```python
from build123d import *

# Parameters (mm, degrees)
SKETCH1_W           = 42
SKETCH1_H           = 42
BOSS_EXTRUDE1_DEPTH = 2
SKETCH2_R           = 2.225
SKETCH2_R_2         = 19
CUT_EXTRUDE1_DEPTH  = 2
FILLET1_R           = 5


with BuildPart() as part:
    # Sketch1 → Boss-Extrude1 (new body)
    with BuildSketch(Plane(origin=(0, 0, 0), x_dir=(1, 0, 0), z_dir=(0, 1, 0))):
        Rectangle(SKETCH1_W, SKETCH1_H)
    extrude(amount=BOSS_EXTRUDE1_DEPTH)

    # Sketch2 → Cut-Extrude1 (cut)
    with BuildSketch(Plane(origin=(0, 2, 0), x_dir=(1, 0, 0), z_dir=(0, 1, 0))):
        with Locations((-16, -16)):
            Circle(SKETCH2_R)
        with Locations((-16, 16)):
            Circle(SKETCH2_R)
        with Locations((16, 16)):
            Circle(SKETCH2_R)
        with Locations((16, -16)):
            Circle(SKETCH2_R)
        Circle(SKETCH2_R_2)
    extrude(amount=-CUT_EXTRUDE1_DEPTH, mode=Mode.SUBTRACT)

    # Fillet1
    fillet1_edges = [part.edges().sort_by_distance(p)[0] for p in [
        (-21, 1, 21),
        (-21, 1, -21),
        (21, 1, -21),
        (21, 1, 21),
    ]]
    fillet(fillet1_edges, radius=FILLET1_R)


solid = part.part
```
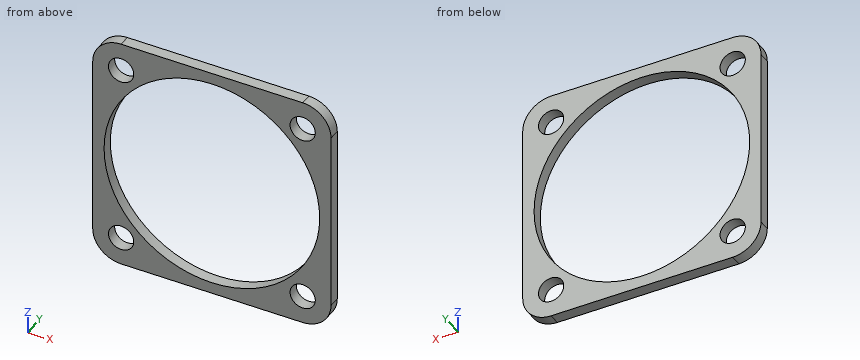
Geometry check sheet. Reference: the model listing, model coordinates, mm. Give positions to 0.01 mm unless a question says otherwise; leave off trailing zeros. Loops run counter-clockwise (first coordinate to the right, second up) from the corner with the lowest first, then second, coordinate; pieces in that order, holes last. Notation, with made-up numbers: M -37.75,85 L -11.75,85 A11 ccw -11.75,96 Z; hole C -12.75,16.25 d4. An arc over 180 degrees is marked long. Answer as CSV lines item,"result".
Item 1: Depth check by flat-ended pin: P1, Ø6, axis at x = 16, z = -16, coming from the +Y side; P2, Ø3.5, axis at x = 16, z = 16, coming from the -Y side. Enter the tip coordinate at first touch or a pass-through.
Values:
P1,"stops at y = 2"
P2,"passes through"
Item 2: Material ranges on line 1 (X direction, y = 1.3, z = 0); line 2 (X direction, y = 1.65, z = 16) (3 decimals), recorded low to high.
Values:
line 1,"x = -21 to -19, 19 to 21"
line 2,"x = -21 to -18.225, -13.775 to -10.247, 10.247 to 13.775, 18.225 to 21"
Item 3: Cross-section at B-B on x = 0. Record the cut outline in (y, z), and give its area (3 significant figures).
Values:
outline,"M 0,-21 L 2,-21 L 2,-19 L 0,-19 Z; M 0,19 L 2,19 L 2,21 L 0,21 Z"
area,"8.00 mm²"
Item 4: Cross-section at D-D on z = -17.5. Record the cut outline in (x, y), and give its area (3 significant figures).
Values:
outline,"M -20.77,0 L -17.64,0 L -17.64,2 L -20.77,2 Z; M -14.36,0 L -7.4,0 L -7.4,2 L -14.36,2 Z; M 7.4,0 L 14.36,0 L 14.36,2 L 7.4,2 Z; M 17.64,0 L 20.77,0 L 20.77,2 L 17.64,2 Z"
area,"40.3 mm²"
Item 5: Cross-section at A-A on z = 5. Record the cut outline in (x, y), and give its area (3 significant figures).
Values:
outline,"M -21,0 L -18.33,0 L -18.33,2 L -21,2 Z; M 18.33,0 L 21,0 L 21,2 L 18.33,2 Z"
area,"10.7 mm²"
Item 6: Cross-section at C-C on y = 0.8. Record the cut outline in (x, z) (3 decimals), and give its area (3 significant figures).
Values:
outline,"M -21,-16 A5 ccw -16,-21 L 16,-21 A5 ccw 21,-16 L 21,16 A5 ccw 16,21 L -16,21 A5 ccw -21,16 Z; hole C 0,0 d38; hole C -16,-16 d4.45; hole C -16,16 d4.45; hole C 16,-16 d4.45; hole C 16,16 d4.45"
area,"546 mm²"
